Source: CAD feature listing. Evaluate the final solid. Frame: model axes, mm. A direction names the side the tool comes from. Give positions to 0.01 mm unless a question says otherwise; leave off trailing zeros.
Solid Edge part; units mm, degrees
sketch "Sketch1" plane through (0, 0, 0) normal (0, 0, 1) x (1, 0, 0)
  line L0 (-20, -20) -> (20, -20)
  line L1 (20, -20) -> (20, 20)
  line L2 (20, 20) -> (-20, 20)
  line L3 (-20, 20) -> (-20, -20)
  dimension "D1" = 20
extrude "Protrusion1" add sketch "Sketch1" along normal blind 10
sketch "Sketch2" plane through (0, 0, 10) normal (0, 0, 1) x (1, 0, 0)
  line L0 (-15, -15) -> (15, -15)
  line L1 (15, -15) -> (15, 15)
  line L2 (15, 15) -> (-15, 15)
  line L3 (-15, 15) -> (-15, -15)
  dimension "D1" = 15
extrude "ExtrudedProtrusion_2" add sketch "Sketch2" along normal blind 6
chamfer "Chamfer_1" distance 5 angle 45 4 edges at (-15, 0, 10) (0, -15, 10) (0, 15, 10) (15, 0, 10)
hole "Hole_1" at (0, 0, 16) direction (0, 0, -1) diameter 5.7 depth 40 tip angle 118 start chamfer 0.6 start chamfer angle 30 end chamfer 0.6 end chamfer angle 30
fillet "Round_1" radius 2 4 edges at (-20, 0, 0) (0, 20, 0) (20, 0, 0) (0, -20, 0)
properties material "Polyethylene, low density"
(1) Reachability of faces 4 (the flat face through (0.2, 15, 15.5)), 5 (the flat face through (15, -0.2, 15.5)), 6 (the flat face through (-15, 0.2, 15.5)) from +Z, -Z, +X, -X, +Y, -Y: full face, straight path, thin tool, end or side. Return the list, or none.
A:
face 4: +Z, +X, -X, +Y
face 5: +Z, +X, +Y, -Y
face 6: +Z, -X, +Y, -Y
(2) First-contact query: pin 1 (3 mm diameter, centred on y = 7, z = 12, fed in from -X); pin 2 (6.5 mm diameter, centred on x = 0, y = 0, fed in from +Z); pin 3 (1 mm diameter, centred on x = 8, z = 13.5, fed in from +Y); pin 4 (8 mm diameter, centred on x = -2, y = 2.5, fed in from -Z). Flat tips, straight axial feed; report the tip coordinate or a pass-through.
A:
pin 1: stops at x = -19.5
pin 2: stops at z = 15.65
pin 3: stops at y = 17
pin 4: stops at z = 0
(3) Ray query, line 1 along X through (y, z) = (0, 5.5); line 2 along X through (y, z) = (0, 12). Return the intervals inside material, ascending.
A:
line 1: x = -20 to -2.85, 2.85 to 20
line 2: x = -18 to -2.85, 2.85 to 18
(4) Mould query, pull axis Y, two halves, no side actions, for faces 1 (the cylindrical face through (1.734, 2.262, 7.903)), 2 (the cylindrical face through (19.43, 0.28, 0.6)), 3 (the flat face through (0, 20, 6)). Classes: pulls with the +Y half, pulls with the -Y half, needs draft (parallel to the pull), parting line crosses it, or undercut.
A:
face 1: undercut
face 2: needs draft
face 3: pulls with the +Y half
